Study the drawing (mm; zero at the part's minimum x, y, z) and answer. A direction names the side the tool comes from. Coordinates: 2 decimals unless noted, no trailing zeros. Loops run counter-clockwise (first coordinate to the right, second up) from the corner with the lowest first, then second, coordinate; pieces in that order, holes last. Notation, with made-up numbers: (45.5, 57) - (87.5, 57) arc R31 ccw to (87.5, 93) - close; hole circle Ø2 at (41, 24). An arc over 180 degrees is marked (long way). Use one line per item in the form item = value.
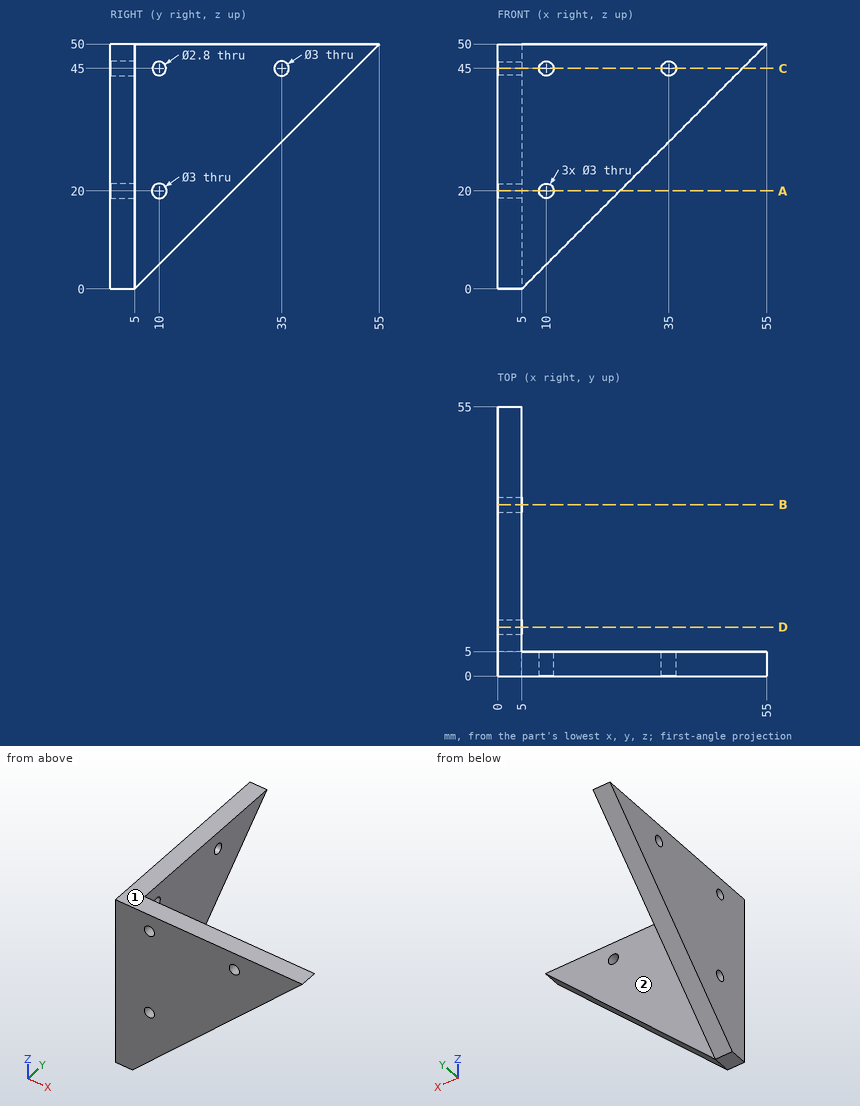
Item 1: The part is cut by section A-A on z = 20. Give the vertices of the cut face in (x, y), plus the area to 3 significant figures.
Results below:
outline = (0, 0) - (8.5, 0) - (8.5, 5) - (5, 5) - (5, 8.5) - (0, 8.5) - close; (0, 11.5) - (5, 11.5) - (5, 25) - (0, 25) - close; (11.5, 0) - (25, 0) - (25, 5) - (11.5, 5) - close
area = 195 mm²
Item 2: Which of the six approach directions +Z, -Z, +X, -X, +Y, -Y give full straight-line access (tool end or side, diameter ignored) to the marked faces 1 and 2?
Results below:
face_1 = +Z, +X, -X, +Y, -Y
face_2 = +Z, -Z, +X, +Y
Item 3: The part is cut by section B-B on y = 35. Give the vertices of the cut face in (x, z), plus the area to 3 significant figures.
Results below:
outline = (0, 30) - (5, 30) - (5, 43.5) - (0, 43.5) - close; (0, 46.5) - (5, 46.5) - (5, 50) - (0, 50) - close
area = 85.0 mm²
Item 4: Each of these flat-tipped pins is pushed along its axis until it touches: P1, Ø2.5, axis at y = 35, z = 45, coming from the +X side; P2, Ø15, axis at y = 22, z = 35.5, coming from the +X side; P3, Ø15, axis at x = 22.5, z = 18.5, coming from the +Y side. Where does it stop, or does it pass through?
Results below:
P1 = through
P2 = 5
P3 = 5
Item 5: The part is cut by section D-D on y = 10. Give the vertices of the cut face in (x, z), plus the area to 3 significant figures.
Results below:
outline = (0, 5) - (5, 5) - (5, 18.5) - (0, 18.5) - close; (0, 21.5) - (5, 21.5) - (5, 43.6) - (0, 43.6) - close; (0, 46.4) - (5, 46.4) - (5, 50) - (0, 50) - close
area = 196 mm²
Item 6: The part is cut by section C-C on z = 45. Give the vertices of the cut face in (x, y), plus the area to 3 significant figures.
Results below:
outline = (0, 0) - (8.5, 0) - (8.5, 5) - (5, 5) - (5, 8.6) - (0, 8.6) - close; (0, 11.4) - (5, 11.4) - (5, 33.5) - (0, 33.5) - close; (0, 36.5) - (5, 36.5) - (5, 50) - (0, 50) - close; (11.5, 0) - (33.5, 0) - (33.5, 5) - (11.5, 5) - close; (36.5, 0) - (50, 0) - (50, 5) - (36.5, 5) - close
area = 416 mm²
Item 7: Find the intervals of material crossed by L1, parallel to X at y = 2.4, z = 45; L2, parallel to Y at x = 3, z = 45; L3, parallel to Y at x = 9.5, z = 37, in increasing order.
Results below:
L1 = 0 to 8.5, 11.5 to 33.5, 36.5 to 50
L2 = 0 to 8.6, 11.4 to 33.5, 36.5 to 50
L3 = 0 to 5
